from build123d import *

# Parameters (mm, degrees)
F1_DEPTH = 6.35
F3_DEPTH = 12.701
F6_R     = 2.54


with BuildPart() as f1:
    # F0 (on Top) → F1 (new body, symmetric)
    with BuildSketch(Plane.XY):
        with BuildLine():
            Line((21.59, 7.62), (-21.59, 7.62))
            ThreePointArc((-21.59, 7.62), (-44.45, 0), (-21.59, -7.62))
            Line((-21.59, -7.62), (21.59, -7.62))
            ThreePointArc((21.59, -7.62), (44.45, 0), (21.59, 7.62))
        make_face()
    extrude(amount=F1_DEPTH, both=True)

    # F4: F3 across plane


with BuildPart() as f3:
    # F2 (on face) → F3 (new body, through all)
    with BuildSketch(Plane.XY.offset(6.35)):
        Polygon((-48.365288, 0), (-43.232644, -8.89), (-32.967356, -8.89), (-27.834712, 0), (-32.967356, 8.89), (-43.232644, 8.89), align=None)
    extrude(amount=-F3_DEPTH)


with BuildPart() as f1_1:
    add(f1.part)
    add(f3.part.mirror(Plane.YZ), mode=Mode.SUBTRACT)

    # F5: cut F3
    add(f3.part, mode=Mode.SUBTRACT)

    # F6
    f6_edges = [f1_1.edges().sort_by_distance(p)[0] for p in [
        (0, -7.62, 6.35),
        (-30.913065, 12.672393, 6.35),
        (-30.913065, -12.672393, 6.35),
        (0, 7.62, 6.35),
        (30.913065, -12.672393, 6.35),
        (30.913065, 12.672393, 6.35),
    ]]
    fillet(f6_edges, radius=F6_R)


solid = f1_1.part
Source: CAD feature listing. Evaluate the final solid. Frame: model axes, mm. A direction names the side the tool comes from. Round coordinates to 2 decimals unless told otherwise and drop trailing zeros. Write each loop counter-clockwise with the first axis right and the second up, starting at its lowest first coordinate (ties: lowest second). Pieces come first, ordered by that corner, then holes. Notation, with made-up numbers: (-25, 60.5) - (1, 60.5) arc R37 cw to (1, 96.5) - close; hole circle Ø1 at (33.25, 74.5). An arc over 180 degrees is marked (long way). Use CSV: the item, a comma, the result in double quotes. Start each with the question number.
(1) Set-up query: faces 4 (the face through (-37, 8.89, 0)), 5 (the face through (0, -7.62, -1)), 6 (the face through (0, 7.62, -1)), 7 (the face through (0.321, -6.856, 5.626)), 8 (the face through (30.44, -4.51, 0.09)). Return all of +Z, -Z, +X, -X, +Y, -Y with unobstructed straight access to the full face (end or side cutting, diameter ignored); none if empty.
(2) Material intervals for probe 1 along Y at (x, z) = (-0.5, 2.5); probe 2 along X at (y, z) = (-8, -2.75); probe 3 along X at (y, z) = (0, -1.75), sorted ascending. Write a range as [from, to].
(3) Mould query, pull axis Y, two halves, no side actions, for faces 1 (the face through (-30.44, -4.51, 0.09)), 2 (the face through (-0.321, 6.896, 5.586)), 3 (the face through (-1, 0, -6.35)). Classes: pulls with the +Y half, pulls with the -Y half, needs draft (parallel to the pull), parting line crosses it, or undercut.
(4) Cut plane D-D, the plane z = 5.25. Return loops of the section in (x, y).
(5) Cut plane B-B, the plane x = -9.5. Return loops of the section in (y, z), and give its area (3 significant figures).
(6) Cut plane A-A, the plane z = -5. Return loops of the section in (x, y).
(7) Cut plane C-C, the plane y = 4. Return loops of the section in (x, z).
(8) First-contact query: pin 1 Ø4 at (x, z) = (36, 0.5) entering from -Y; pin 2 Ø4 at (x, z) = (-36.5, -2) entering from +Y; pin 3 Ø3 at (x, z) = (-7, 0) entering from +Y. Flat tips, straight axial feed; report the tip coordinate or a pass-through.
Geometry says:
1,face 4,"+Z, -Z, -X"
1,face 5,"+Z, -Z, -Y"
1,face 6,"+Z, -Z, +Y"
1,face 7,"+Z, -Y"
1,face 8,"+Z, -Z, +X"
2,probe 1,"[-7.62, 7.62]"
2,probe 2,"[-32.45, -21.89], [21.89, 32.45]"
2,probe 3,"[-27.83, 27.83]"
3,face 1,"undercut"
3,face 2,"pulls with the +Y half"
3,face 3,"needs draft"
4,outline,"(-40.18, -8.89) arc R12.25 ccw to (-21.82, -7.17) - (21.82, -7.17) arc R12.25 ccw to (40.18, -8.89) - (32.97, -8.89) - (27.83, 0) - (32.97, 8.89) - (40.18, 8.89) arc R12.25 ccw to (21.82, 7.17) - (-21.82, 7.17) arc R12.25 ccw to (-40.18, 8.89) - (-32.97, 8.89) - (-27.83, 0) - (-32.97, -8.89) - close"
5,outline,"(-7.62, -6.35) - (7.62, -6.35) - (7.62, 3.81) arc R2.54 ccw to (5.08, 6.35) - (-5.08, 6.35) arc R2.54 ccw to (-7.62, 3.81) - close"
5,area,"191 mm²"
6,outline,"(-40.82, -8.89) arc R12.7 ccw to (-21.59, -7.62) - (21.59, -7.62) arc R12.7 ccw to (40.82, -8.89) - (32.97, -8.89) - (27.83, 0) - (32.97, 8.89) - (40.82, 8.89) arc R12.7 ccw to (21.59, 7.62) - (-21.59, 7.62) arc R12.7 ccw to (-40.82, 8.89) - (-32.97, 8.89) - (-27.83, 0) - (-32.97, -8.89) - close"
7,outline,"(-30.14, -6.35) - (30.14, -6.35) - (30.14, 6.35) - (-30.14, 6.35) - close"
8,pin 1,"y = -12.5"
8,pin 2,"y = 12.4"
8,pin 3,"y = 7.62"
